```python
from build123d import *

# Parameters (mm, degrees)
SKETCH1_W            = 6.2738
SKETCH1_H            = 6.35
BOSS_EXTRUDE1_DEPTH  = 3.175
BOSS_EXTRUDE2_DEPTH  = 5.08
SKETCH3_W            = 6.35
SKETCH3_H            = 3.175
BOSS_EXTRUDE3_DEPTH  = 1.1938
SKETCH4_W            = 0.889
SKETCH4_H            = 0.635
CUT_EXTRUDE1_DEPTH   = 10.884786195
SKETCH5_W            = 0.635
SKETCH5_H            = 0.635
BOSS_EXTRUDE4_DEPTH  = 3.683
SKETCH6_W            = 0.635
SKETCH6_H            = 0.635
BOSS_EXTRUDE5_DEPTH  = 6.4389
SKETCH7_W            = 0.889
SKETCH7_H            = 0.635
CUT_EXTRUDE2_DEPTH   = 10.884786195
SKETCH8_W            = 0.635
SKETCH8_H            = 0.635
BOSS_EXTRUDE6_DEPTH  = 3.683
SKETCH9_W            = 0.635
SKETCH9_H            = 0.635
BOSS_EXTRUDE7_DEPTH  = 6.4389
SKETCH10_W           = 0.889
SKETCH10_H           = 0.635
CUT_EXTRUDE3_DEPTH   = 10.884786195
SKETCH11_W           = 0.635
SKETCH11_H           = 0.635
BOSS_EXTRUDE8_DEPTH  = 3.683
SKETCH12_W           = 0.635
SKETCH12_H           = 0.635
BOSS_EXTRUDE9_DEPTH  = 6.4389
SKETCH13_W           = 0.635
SKETCH13_H           = 0.635
BOSS_EXTRUDE10_DEPTH = 6.7056
SKETCH14_W           = 0.635
SKETCH14_H           = 0.635
BOSS_EXTRUDE11_DEPTH = 6.7056
SKETCH15_W           = 0.635
SKETCH15_H           = 0.635
BOSS_EXTRUDE12_DEPTH = 6.7056
CUT_EXTRUDE4_DEPTH   = 4.572
CUT_EXTRUDE5_DEPTH   = 4.572
FILLET1_R            = 1.1684
FILLET2_R            = 1.8034


with BuildPart() as part:
    # Sketch1 → Boss-Extrude1 (new body)
    with BuildSketch(Plane.XZ.offset(1.5875)):
        with Locations((-0.5969, 0)):
            Rectangle(SKETCH1_W, SKETCH1_H)
    extrude(amount=-BOSS_EXTRUDE1_DEPTH)

    # Sketch2 → Boss-Extrude2 (add)
    with BuildSketch(Plane(origin=(2.54, 0, 0), x_dir=(0, 0, -1), z_dir=(1, 0, 0))):
        Polygon((1.3843, 3.3655), (2.286, 2.6035), (2.286, 1.5875), (3.175, 1.5875), (3.175, 6.5913), (2.457539437, 6.5913), (1.3843, 5.3213), align=None)
    extrude(amount=-BOSS_EXTRUDE2_DEPTH)

    # Sketch3 → Boss-Extrude3 (add)
    with BuildSketch(Plane(origin=(2.54, 0, 0), x_dir=(0, 0, -1), z_dir=(1, 0, 0))):
        Rectangle(SKETCH3_W, SKETCH3_H)
    extrude(amount=BOSS_EXTRUDE3_DEPTH)

    # Sketch4 → Cut-Extrude1 (cut, through all)
    with BuildSketch(Plane.XY.offset(3.175)):
        with Locations((0, -1.27)):
            Rectangle(SKETCH4_W, SKETCH4_H)
    extrude(amount=-CUT_EXTRUDE1_DEPTH, mode=Mode.SUBTRACT)

    # Sketch5 → Boss-Extrude4 (add)
    with BuildSketch(Plane.XZ.offset(0.9525)):
        Rectangle(SKETCH5_W, SKETCH5_H)
    extrude(amount=BOSS_EXTRUDE4_DEPTH)

    # Sketch6 → Boss-Extrude5 (add)
    with BuildSketch(Plane.XY.offset(0.3175)):
        with Locations((0, -4.318)):
            Rectangle(SKETCH6_W, SKETCH6_H)
    extrude(amount=BOSS_EXTRUDE5_DEPTH)

    # Sketch7 → Cut-Extrude2 (cut, through all)
    with BuildSketch(Plane.XY.offset(3.175)):
        with Locations((-2.54, -1.27)):
            Rectangle(SKETCH7_W, SKETCH7_H)
    extrude(amount=-CUT_EXTRUDE2_DEPTH, mode=Mode.SUBTRACT)

    # Sketch8 → Boss-Extrude6 (add)
    with BuildSketch(Plane.XZ.offset(0.9525)):
        with Locations((-2.54, 0)):
            Rectangle(SKETCH8_W, SKETCH8_H)
    extrude(amount=BOSS_EXTRUDE6_DEPTH)

    # Sketch9 → Boss-Extrude7 (add)
    with BuildSketch(Plane.XY.offset(0.3175)):
        with Locations((-2.54, -4.318)):
            Rectangle(SKETCH9_W, SKETCH9_H)
    extrude(amount=BOSS_EXTRUDE7_DEPTH)

    # Sketch10 → Cut-Extrude3 (cut, through all)
    with BuildSketch(Plane.XY.offset(3.175)):
        with Locations((2.54, -1.27)):
            Rectangle(SKETCH10_W, SKETCH10_H)
    extrude(amount=-CUT_EXTRUDE3_DEPTH, mode=Mode.SUBTRACT)

    # Sketch11 → Boss-Extrude8 (add)
    with BuildSketch(Plane.XZ.offset(0.9525)):
        with Locations((2.54, 0)):
            Rectangle(SKETCH11_W, SKETCH11_H)
    extrude(amount=BOSS_EXTRUDE8_DEPTH)

    # Sketch12 → Boss-Extrude9 (add)
    with BuildSketch(Plane.XY.offset(0.3175)):
        with Locations((2.54, -4.318)):
            Rectangle(SKETCH12_W, SKETCH12_H)
    extrude(amount=BOSS_EXTRUDE9_DEPTH)

    # Sketch13 → Boss-Extrude10 (add)
    with BuildSketch(Plane(origin=(0, 1.5875, 0), x_dir=(-1, 0, 0), z_dir=(0, 1, 0))):
        with Locations((2.54, 0)):
            Rectangle(SKETCH13_W, SKETCH13_H)
    extrude(amount=BOSS_EXTRUDE10_DEPTH)

    # Sketch14 → Boss-Extrude11 (add)
    with BuildSketch(Plane(origin=(0, 1.5875, 0), x_dir=(-1, 0, 0), z_dir=(0, 1, 0))):
        Rectangle(SKETCH14_W, SKETCH14_H)
    extrude(amount=BOSS_EXTRUDE11_DEPTH)

    # Sketch15 → Boss-Extrude12 (add)
    with BuildSketch(Plane(origin=(0, 1.5875, 0), x_dir=(-1, 0, 0), z_dir=(0, 1, 0))):
        with Locations((-2.54, 0)):
            Rectangle(SKETCH15_W, SKETCH15_H)
    extrude(amount=BOSS_EXTRUDE12_DEPTH)

    # Sketch16 → Cut-Extrude4 (cut)
    with BuildSketch(Plane(origin=(0, 0, -2.286), x_dir=(-1, 0, 0), z_dir=(0, 0, -1))):
        Polygon((3.7338, 0.762), (3.4798, 0.635), (3.4798, -0.127), (3.7338, -0.254), align=None)
    extrude(amount=-CUT_EXTRUDE4_DEPTH, mode=Mode.SUBTRACT)

    # Sketch17 → Cut-Extrude5 (cut)
    with BuildSketch(Plane(origin=(0, 0, -2.286), x_dir=(-1, 0, 0), z_dir=(0, 0, -1))):
        Polygon((-3.7338, -0.254), (-3.4798, -0.127), (-3.4798, 0.635), (-3.7338, 0.762), align=None)
    extrude(amount=-CUT_EXTRUDE5_DEPTH, mode=Mode.SUBTRACT)

    # Fillet1
    fillet1_edges = [part.edges().sort_by_distance(p)[0] for p in [
        (-2.54, -4.0005, 0.3175),
        (2.54, -4.0005, 0.3175),
        (0, -4.0005, 0.3175),
    ]]
    fillet(fillet1_edges, radius=FILLET1_R)

    # Fillet2
    fillet2_edges = [part.edges().sort_by_distance(p)[0] for p in [
        (-2.54, -4.6355, -0.3175),
        (2.54, -4.6355, -0.3175),
        (0, -4.6355, -0.3175),
    ]]
    fillet(fillet2_edges, radius=FILLET2_R)


solid = part.part
```
Check sheet for the modelled part. Datum: model origin and axes. Units: mm. A direction names the side the tool comes from. Coordinates: 2 decimals unless noted, no trailing zeros. Write each loop counter-clockwise with the first axis right and the second up, starting at its lowest first coordinate (ties: lowest second). Pieces come first, ordered by that corner, then holes. Notation, with made-up numbers: M 25.25,66.25 L 36.25,66.25 A10 cw 36.25,83.25 Z; hole C -38.75,54.25 d9. An arc over 180 degrees is marked long. Write item = value, one per line. Start each with the question number.
1. Mould release check, pull along X, two halves, no side actions. Record for faces 1 (the flat face through (-2.5, -0.952, -0.7)), 2 (the flat face through (0.318, -4.2, 2.4)), 3 (the flat face through (2.54, 4, -2)), 4 (the flat face through (0, 4, -1.384)): pulls with the +X half, pulls with the -X half, needs draft (parallel to the pull), parting line crosses it, or undercut.
2. Tool access check on faces 5 (the flat face through (0.04, 2.99, -1.83)), 6 (the flat face through (-2.222, -4.2, 2.4)), 7 (the flat face through (0.04, 5.97, -1.93)), 8 (the flat face through (0, 0, 3.175)), 9 (the cylindrical face through (2.54, -3.67, 0.67)). Record the directions out of +Z, -Z, +X, -X, +Y, -Y that give a thin tool (end or side, any length) a straight path to the whole face; none if there is none.
3. Sectioned sample at B-B (z = 3.5). Record the cut outline in (x, y), then the cut area to 3 significant figures.
4. Go/stop test with flat-tipped pins: pin 1 (1.8 mm diameter, centred on x = -1, z = 0, fed in from -Y); pin 2 (1.4 mm diameter, centred on y = 4.5, z = -2, fed in from +X); pin 3 (1.5 mm diameter, centred on y = 5.5, z = -1.5, fed in from -X); pin 4 (1 mm diameter, centred on y = -1.5, z = 4.5, fed in from +X). Record where each tip stops, or that it passes through.
5. Thickness scan on probe 1 along X at (y, z) = (-1.25, 2.75); probe 2 along Y at (x, z) = (0.5, 0.25); probe 3 along Z at (x, y) = (1.5, 2.25) (3 decimals). Record the ranges inside material, lowest first.
6. Sectioned sample at A-A (y = 5). Record the cut outline in (x, z) (1 decimal), then the cut area to 3 significant figures.
7. Sectioned sample at C-C (y = -2.5). Record the cut outline in (x, z), then the cut area to 3 significant figures.
The answers:
q1.face_1 = undercut
q1.face_2 = undercut
q1.face_3 = pulls with the +X half
q1.face_4 = needs draft
q2.face_5 = +X, -X
q2.face_6 = +Z, -Z, -Y
q2.face_7 = +X, -X, +Y
q2.face_8 = +Z, +X, -X, +Y
q2.face_9 = +Z, +X, -X
q3.outline = M -2.86,-4.64 L -2.22,-4.64 L -2.22,-4 L -2.86,-4 Z; M -0.32,-4.64 L 0.32,-4.64 L 0.32,-4 L -0.32,-4 Z; M 2.22,-4.64 L 2.86,-4.64 L 2.86,-4 L 2.22,-4 Z
q3.area = 1.21 mm²
q4.pin_1 = -4.4
q4.pin_2 = 2.54
q4.pin_3 = -2.54
q4.pin_4 = through
q5.probe_1 = -3.73 to -2.98, -2.1 to -0.44, 0.44 to 2.1, 2.98 to 3.73
q5.probe_2 = -1.59 to 1.59
q5.probe_3 = -3.175 to -2.286
q6.outline = M -2.9,-0.3 L -2.2,-0.3 L -2.2,0.3 L -2.9,0.3 Z; M -2.5,-3.2 L 2.5,-3.2 L 2.5,-1.4 L -2.5,-1.4 Z; M -0.3,-0.3 L 0.3,-0.3 L 0.3,0.3 L -0.3,0.3 Z; M 2.2,-0.3 L 2.9,-0.3 L 2.9,0.3 L 2.2,0.3 Z
q6.area = 10.3 mm²
q7.outline = M -2.86,-0.32 L -2.22,-0.32 L -2.22,0.32 L -2.86,0.32 Z; M -0.32,-0.32 L 0.32,-0.32 L 0.32,0.32 L -0.32,0.32 Z; M 2.22,-0.32 L 2.86,-0.32 L 2.86,0.32 L 2.22,0.32 Z
q7.area = 1.21 mm²
